from build123d import *

# Parameters (mm, degrees)
F0_R     = 7.5
F1_DEPTH = 0.7
F2_R     = 0.183
F3_DEPTH = 50


with BuildPart() as f1:
    # F0 (on Top) → F1 (new body)
    with BuildSketch(Plane.XY):
        Circle(F0_R)
    extrude(amount=F1_DEPTH)

    # F2 (on Top) → F3 (join)
    with BuildSketch(Plane.XY):
        with Locations((-2.734368, 2.716938)):
            Circle(F2_R)
        with Locations((2.83951, 2.785288)):
            Circle(F2_R)
        with Locations((2.876553, -2.831199)):
            Circle(F2_R)
        with Locations((-2.841227, -2.724453)):
            Circle(F2_R)
    extrude(amount=F3_DEPTH)


solid = f1.part
Build history of the part. All positions in model axes, mm. Give positions to 0.01 mm unless a question says otherwise; leave off trailing zeros. Loops run counter-clockwise (first coordinate to the right, second up) from the corner with the lowest first, then second, coordinate; pieces in that order, holes last. Notation, with made-up numbers: (-6, -4) -> (38, -4) arc R32 ccw to (38, 26) -> close; hole circle Ø11 at (-11.75, 6.5). An arc over 180 degrees is marked (long way). Answer in a Markdown table with one row per item.
Item 1: Slice it at C-C on z = 3.5. Write the cut outline in (x, y).
Findings below:
| item | result |
|---|---|
| outline | circle Ø0.37 at (-2.84, -2.72); circle Ø0.37 at (-2.73, 2.72); circle Ø0.37 at (2.84, 2.79); circle Ø0.37 at (2.88, -2.83) |
Item 2: Flat gauge pins, fed straight in: P1, Ø5, axis at y = 3.5, z = 13.5, coming from the +X side; P2, Ø5, axis at y = -3.5, z = 36.5, coming from the -X side; P3, Ø5, axis at x = 4.5, y = -4, coming from the -Z side; P4, Ø1, axis at x = -5.5, y = -3.5, coming from the +Z side. Where does each tip first touch, or does it go through?
Findings below:
| item | result |
|---|---|
| P1 | stops at x = 3.02 |
| P2 | stops at x = -3.02 |
| P3 | stops at z = 0 |
| P4 | stops at z = 0.7 |
Item 3: Probe line 1 along X through (y, z) = (2.75, 37); line 2 along Z through (x, y) = (-3.25, 5.5). List the from-to ranges inside material, lowest first. Write a range as [from, to].
Findings below:
| item | result |
|---|---|
| line 1 | x = [-2.91, -2.55], [2.66, 3.02] |
| line 2 | z = [0, 0.7] |
Item 4: Mould opens along Z. For faces 1 (the flat face through (0, 0, 0.7)), 2 (the flat face through (0, 0, 0)), 3 (the cylindrical face through (-7.493, 0.33, 0.345)) say: pulls with the +Z half, pulls with the -Z half, needs draft (parallel to the pull), parting line crosses it, or undercut.
Findings below:
| item | result |
|---|---|
| face 1 | pulls with the +Z half |
| face 2 | pulls with the -Z half |
| face 3 | needs draft |
Item 5: Slice it at A-A on y = 0. Write the cut outline in (x, z), plus the area to 3 significant figures.
Findings below:
| item | result |
|---|---|
| outline | (-7.5, 0) -> (7.5, 0) -> (7.5, 0.7) -> (-7.5, 0.7) -> close |
| area | 10.5 mm² |
